from build123d import *

# Parameters (mm, degrees)
F1_DEPTH       = 28.1119
F1_TAPER       = -20
F3_D           = 5
F3_CBORE_D     = 10
F3_CBORE_DEPTH = 5


with BuildPart() as f1:
    # F0 (on Front) → F1 (new body)
    with BuildSketch(Plane.XZ):
        Polygon((-37.6286933092, 1.1261076269), (-25.476778123, 8.0027721288), (-18.3912431181, 20.0340958739), (-18.270651677, 33.9962953808), (-25.1473161789, 46.148210567), (-37.178639924, 53.2337455719), (-51.1408394309, 53.354337013), (-63.2927546171, 46.4776725111), (-70.378289622, 34.446348766), (-70.4988810631, 20.4841492591), (-63.6222165612, 8.3322340729), (-51.5908928161, 1.246699068), align=None)
    extrude(amount=F1_DEPTH, taper=F1_TAPER)

    # F3 (through all)
    with Locations(Plane.XZ.offset(28.1119)):
        with Locations((-77.7391013168, 17.3710930631), (-65.139479872, 55.7104988926), (-24.7830409778, 55.5750747702), (-12.4410115211, 17.1519722301), (-45.0544580817, 27.8698503971)):
            CounterBoreHole(F3_D / 2, F3_CBORE_D / 2, F3_CBORE_DEPTH)


solid = f1.part
Source: CAD feature listing. Evaluate the final solid. Frame: model axes, mm. A direction names the side the tool comes from. Round coordinates to 2 decimals unless told otherwise and drop trailing zeros.
Q1. First-contact query: P1, Ø3.5, axis at x = -14, z = 15.5, coming from the -Y side; P2, Ø10, axis at x = -38.5, y = -15, coming from the +Z side; P3, Ø4, axis at x = -72, y = -12.5, coming from the +Z side. Flat tips, straight axial feed; report the tip coordinate or a pass-through.
Q2. Access query for faces 1 (the face through (-48.74, -25.65, 31.25)), 2 (the face through (-50, 0, 25)). Directions: +Z, -Z, +X, -X, +Y, -Y. A direction counts if a zero-diameter tool reaches every point of the face in a straight line with its end or side. Return the directions, or none.
Q3. Ray query, line 1 (Z direction, x = -44.5, y = -22.5); line 2 (X direction, y = -5.5, z = 28.5); line 3 (X direction, y = -2.5, z = 28). Return the intervals inside material, ascending.
Solutions:
1. P1: stops at y = -23.11
1. P2: stops at z = 60.53
1. P3: stops at z = 44.34
2. face 1: -Y
2. face 2: +Z, -Z, +X, -X, +Y
3. line 1: z = -7 to 25.43, 30.31 to 61.49
3. line 2: x = -72.43 to -47.47, -42.64 to -16.32
3. line 3: x = -71.34 to -47.55, -42.56 to -17.41
